Here's how the part is built. I have some questions about the finished solid (model axes, mm). A direction names the side the tool comes from. Coordinates: 2 decimals unless noted, no trailing zeros. Loops run counter-clockwise (first coordinate to the right, second up) from the corner with the lowest first, then second, coordinate; pieces in that order, holes last.
from build123d import *

# Parameters (mm, degrees)
SKETCH1_W           = 210
SKETCH1_H           = 210
MAINEXTRUDE_DEPTH   = 4
SKETCH1_6_R         = 1.5
SCREWHOLES_DEPTH    = 4
ROUNDEDCORNERS_R    = 10
SKETCH4_W           = 140
SKETCH4_H           = 14
SKETCH4_W_2         = 136
SKETCH4_H_2         = 10
TRENCH_WALLS_DEPTH  = 10
SKETCH3_W           = 136
SKETCH3_H           = 10
TRENCH_DEPTH        = 12
SKETCH6_W           = 140
SKETCH6_H           = 14
TRENCH_BOTTOM_DEPTH = 2


with BuildPart() as part:
    # Sketch1 → MainExtrude (new body)
    with BuildSketch(Plane(origin=(0, 0, 0), x_dir=(1, 0, 0), z_dir=(0, 1, 0))):
        Rectangle(SKETCH1_W, SKETCH1_H)
    extrude(amount=MAINEXTRUDE_DEPTH)

    # Sketch1<6> → ScrewHoles (cut)
    with BuildSketch(Plane(origin=(0, 0, 0), x_dir=(1, 0, 0), z_dir=(0, 1, 0))):
        with Locations((-99.833273811, 99.833273811)):
            Circle(SKETCH1_6_R)
        with Locations((-99.833273811, -99.833273811)):
            Circle(SKETCH1_6_R)
        with Locations((99.833273811, -99.833273811)):
            Circle(SKETCH1_6_R)
        with Locations((99.833273811, 99.833273811)):
            Circle(SKETCH1_6_R)
    extrude(amount=SCREWHOLES_DEPTH, mode=Mode.SUBTRACT)

    # RoundedCorners
    roundedcorners_edges = [part.edges().sort_by_distance(p)[0] for p in [
        (-105, 2, -105),
        (-105, 2, 105),
        (105, 2, 105),
        (105, 2, -105),
    ]]
    fillet(roundedcorners_edges, radius=ROUNDEDCORNERS_R)

    # Sketch4 → Trench Walls (add)
    with BuildSketch(Plane(origin=(0, 0, 0), x_dir=(1, 0, 0), z_dir=(0, 1, 0))):
        with Locations((0, 56)):
            Rectangle(SKETCH4_W, SKETCH4_H)
        with Locations((0, 56)):
            Rectangle(SKETCH4_W_2, SKETCH4_H_2, mode=Mode.SUBTRACT)
        with Locations((0, 39)):
            Rectangle(SKETCH4_W, SKETCH4_H)
        with Locations((0, 39)):
            Rectangle(SKETCH4_W_2, SKETCH4_H_2, mode=Mode.SUBTRACT)
        with Locations((0, 22)):
            Rectangle(SKETCH4_W, SKETCH4_H)
        with Locations((0, 22)):
            Rectangle(SKETCH4_W_2, SKETCH4_H_2, mode=Mode.SUBTRACT)
        with Locations((0, 5)):
            Rectangle(SKETCH4_W, SKETCH4_H)
        with Locations((0, 5)):
            Rectangle(SKETCH4_W_2, SKETCH4_H_2, mode=Mode.SUBTRACT)
        with Locations((0, -12)):
            Rectangle(SKETCH4_W, SKETCH4_H)
        with Locations((0, -12)):
            Rectangle(SKETCH4_W_2, SKETCH4_H_2, mode=Mode.SUBTRACT)
        with Locations((0, -29)):
            Rectangle(SKETCH4_W, SKETCH4_H)
        with Locations((0, -29)):
            Rectangle(SKETCH4_W_2, SKETCH4_H_2, mode=Mode.SUBTRACT)
        with Locations((0, -46)):
            Rectangle(SKETCH4_W, SKETCH4_H)
        with Locations((0, -46)):
            Rectangle(SKETCH4_W_2, SKETCH4_H_2, mode=Mode.SUBTRACT)
    extrude(amount=-TRENCH_WALLS_DEPTH)

    # Sketch3 → Trench (cut)
    with BuildSketch(Plane(origin=(0, 0, 0), x_dir=(1, 0, 0), z_dir=(0, 1, 0))):
        with Locations((0, 56)):
            Rectangle(SKETCH3_W, SKETCH3_H)
        with Locations((0, 39)):
            Rectangle(SKETCH3_W, SKETCH3_H)
        with Locations((0, 22)):
            Rectangle(SKETCH3_W, SKETCH3_H)
        with Locations((0, 5)):
            Rectangle(SKETCH3_W, SKETCH3_H)
        with Locations((0, -12)):
            Rectangle(SKETCH3_W, SKETCH3_H)
        with Locations((0, -29)):
            Rectangle(SKETCH3_W, SKETCH3_H)
        with Locations((0, -46)):
            Rectangle(SKETCH3_W, SKETCH3_H)
    extrude(amount=TRENCH_DEPTH, mode=Mode.SUBTRACT)

    # Sketch6 → Trench Bottom (add)
    with BuildSketch(Plane.XZ.offset(10)):
        with Locations((0, -56)):
            Rectangle(SKETCH6_W, SKETCH6_H)
        with Locations((0, -39)):
            Rectangle(SKETCH6_W, SKETCH6_H)
        with Locations((0, -22)):
            Rectangle(SKETCH6_W, SKETCH6_H)
        with Locations((0, -5)):
            Rectangle(SKETCH6_W, SKETCH6_H)
        with Locations((0, 12)):
            Rectangle(SKETCH6_W, SKETCH6_H)
        with Locations((0, 29)):
            Rectangle(SKETCH6_W, SKETCH6_H)
        with Locations((0, 46)):
            Rectangle(SKETCH6_W, SKETCH6_H)
    extrude(amount=TRENCH_BOTTOM_DEPTH)


solid = part.part
Q1. We'd pull the mould along Z, two halves only. Please class faces 1 (the flat face through (-1, -6, 5)), 2 (the flat face through (-1, -12, 46)), 3 (the flat face through (68, -3, -39)): pulls with the +Z half, pulls with the -Z half, needs draft (parallel to the pull), parting line crosses it, or undercut.
Q2. Suppose I cut it at C-C on x = -92. Write out the boundary of the cut face in (y, z), and give its area (3 significant figures).
Q3. Please list where these lines run through material, in increasing order: probe 1 along X at (y, z) = (-8.5, 33); probe 2 along Y at (x, z) = (39, 87); probe 3 along Y at (x, z) = (-65.5, -52).
Q4. Suppose I cut it at A-A on z = -6. Write out the boundary of the cut face in (x, y).
Q5. Suppose I cut it at D-D on z = -77.5. Write out the boundary of the cut face in (x, y), and give its area (3 significant figures).
Q6. Suppose I cut it at B-B on y = -5.75. State how many separate pieces and enclosed holes the cut face has, and give its area (3 significant figures).
Q7. Will these pins go through, and if not, where does the flat tip stop? P1, Ø2.5, axis at x = 99.83, z = -99.83, coming from the -Y side; P2, Ø9.5, axis at x = 3, y = -5, coming from the -Z side; P3, Ø3.5, axis at x = -99.83, z = 99.83, coming from the -Y side; P4, Ø3.5, axis at x = 6.5, y = -6, coming from the +Z side.
Q8. For faces 4 (the flat face through (-68, -3, 12)), 5 (the flat face through (-1, -6, -29)), 6 (the flat face through (70, -6, 12)), which set-ups out of +Z, -Z, +X, -X, +Y, -Y let a thin tool reach every point of the face, with its end or its side?
Check values:
1. face 1: undercut
1. face 2: needs draft
1. face 3: undercut
2. outline: (0, -105) - (4, -105) - (4, 105) - (0, 105) - close
2. area: 840 mm2
3. probe 1: x = -70 to -68, 68 to 70
3. probe 2: y = 0 to 4
3. probe 3: y = -12 to -10
4. outline: (-105, 0) - (-70, 0) - (-70, -12) - (70, -12) - (70, 0) - (105, 0) - (105, 4) - (68, 4) - (68, -10) - (-68, -10) - (-68, 4) - (-105, 4) - close
5. outline: (-105, 0) - (105, 0) - (105, 4) - (-105, 4) - close
5. area: 840 mm2
6. separate pieces: 7
6. enclosed holes: 7
6. area: 4,200 mm2
7. P1: passes through
7. P2: stops at z = -63
7. P3: stops at y = 0
7. P4: stops at z = 53
8. face 4: +Y
8. face 5: +X, -X, -Y
8. face 6: +Z, -Z, +X, -Y
